Could you check a few things on this model? Use its own coordinates, in mm. A direction names the side the tool comes from. Give positions to 0.01 mm unless a question says otherwise; leave off trailing zeros. Loops run counter-clockwise (first coordinate to the right, second up) from the corner with the lowest first, then second, coordinate; pieces in that order, holes last. Notation, with made-up numbers: (7, 9.5) - (29, 9.5) arc R10 ccw to (29, 16.5) - close; hole circle Ø5 at (63, 2.5). An arc over 180 degrees is marked (long way). Write each question's results on one line, items separated by ' | '. Start each with the question number.
1) If I drill on probe 1 along Y at (x, z) = (0, -2.25); probe 2 along Y at (x, z) = (4.5, -1.75); probe 3 along Y at (x, z) = (0, -15.25), over which ranges is the centre line in solid material (lowest first)? Write a range as [from, to].
2) I'm going to push flat-ended pins straight in: pin 1 (3.5 mm diameter, centred on x = -1, z = -13.5, fed in from -Y); pin 2 (4 mm diameter, centred on y = 5.5, z = -5.5, fed in from -X); pin 3 (1.5 mm diameter, centred on y = 4, z = -3, fed in from +X); pin 4 (9 mm diameter, centred on x = -2.5, y = 1, fed in from -Z). Where does each tip first touch, or does it pass through?
3) I want a section at A-A, the plane z = -6. Write out the boundary of the cut face in (x, y), and give its area (3 significant figures).
4) On a 3-axis mill with a long thin cutter (end or side, diameter ignored), from which of +Z, -Z, +X, -X, +Y, -Y can I reach the whole of each face in a straight line? I mean faces 4 (the face through (5.04, 5.08, -15)), 5 (the face through (0, 2, -6.5)), 6 (the face through (4, -6, 1)). Say none if no direction works.
5) If we mould it in two halves opening along X, with no side actions, what happens to faces 1 (the face through (-0.1, 1.56, -3.03)), 2 (the face through (7.327, -4.309, -13.521)), 3 (the face through (0, -8.5, -14))? For each: +X half, -X half, draft (parallel to the pull), parting line (faces both ways), or undercut.
6) I want a section at B-B, the plane z = -12.75. Write out the boundary of the cut face in (x, y), and give its area (3 significant figures).
from build123d import *

# Parameters (mm, degrees)
SKETCH1_R          = 9
EXTRUDE1_DEPTH     = 2
SKETCH4_R          = 7
EXTRUDE2_DEPTH     = 16
SKETCH2_R          = 5.5
CUT_EXTRUDE1_DEPTH = 10
SKETCH3_R          = 8.25
SKETCH3_R_2        = 7
CUT_EXTRUDE2_DEPTH = 1
SKETCH5_R          = 5
EXTRUDE3_DEPTH     = 8.5
SKETCH6_R          = 0.45
CUT_EXTRUDE3_DEPTH = 7
CHAMFER2_SIZE      = 0.15
CHAMFER1_SIZE      = 0.2
SKETCH7_R          = 5.5
CUT_EXTRUDE4_DEPTH = 1
CHAMFER3_SIZE      = 0.5
EXTRUDE4_DEPTH     = 3


with BuildPart() as part:
    # Sketch1 → Extrude1 (new body)
    with BuildSketch(Plane.XY):
        Circle(SKETCH1_R)
    extrude(amount=EXTRUDE1_DEPTH)

    # Sketch4 → Extrude2 (add)
    with BuildSketch(Plane(origin=(0, 0, 0), x_dir=(-1, 0, 0), z_dir=(0, 0, -1))):
        Circle(SKETCH4_R)
    extrude(amount=EXTRUDE2_DEPTH)

    # Sketch2 → Cut-Extrude1 (cut)
    with BuildSketch(Plane.XY.offset(2)):
        Circle(SKETCH2_R)
    extrude(amount=-CUT_EXTRUDE1_DEPTH, mode=Mode.SUBTRACT)

    # Sketch3 → Cut-Extrude2 (cut)
    with BuildSketch(Plane(origin=(0, 0, 0), x_dir=(-1, 0, 0), z_dir=(0, 0, -1))):
        Circle(SKETCH3_R)
        Circle(SKETCH3_R_2, mode=Mode.SUBTRACT)
    extrude(amount=-CUT_EXTRUDE2_DEPTH, mode=Mode.SUBTRACT)

    # Sketch5 → Extrude3 (add)
    with BuildSketch(Plane.XY.offset(-8)):
        Circle(SKETCH5_R)
    extrude(amount=EXTRUDE3_DEPTH)

    # Sketch6 → Cut-Extrude3 (cut)
    with BuildSketch(Plane.XY.offset(0.5)):
        with Locations((0, 2)):
            Circle(SKETCH6_R)
        with Locations((0, -2)):
            Circle(SKETCH6_R)
        with Locations((2, 0)):
            Circle(SKETCH6_R)
        with Locations((-2, 0)):
            Circle(SKETCH6_R)
    extrude(amount=-CUT_EXTRUDE3_DEPTH, mode=Mode.SUBTRACT)

    # Chamfer2
    chamfer2_edges = [part.edges().sort_by_distance(p)[0] for p in [
        (-5, 0, 0.5),
        (-0.45, 2, 0.5),
        (-0.45, -2, 0.5),
        (1.55, 0, 0.5),
        (-2.45, 0, 0.5),
    ]]
    chamfer(chamfer2_edges, length=CHAMFER2_SIZE)

    # Chamfer1
    chamfer1_edges = [part.edges().sort_by_distance(p)[0] for p in [
        (-5.5, 0, 2),
        (-9, 0, 2),
    ]]
    chamfer(chamfer1_edges, length=CHAMFER1_SIZE)

    # Sketch7 → Cut-Extrude4 (cut)
    with BuildSketch(Plane(origin=(0, 0, -16), x_dir=(-1, 0, 0), z_dir=(0, 0, -1))):
        Circle(SKETCH7_R)
    extrude(amount=-CUT_EXTRUDE4_DEPTH, mode=Mode.SUBTRACT)

    # Chamfer3
    chamfer3_edges = [part.edges().sort_by_distance(p)[0] for p in [
        (7, 0, -16),
    ]]
    chamfer(chamfer3_edges, length=CHAMFER3_SIZE)

    # Sketch8 → Extrude4 (add)
    with BuildSketch(Plane(origin=(0, 0, -15), x_dir=(-1, 0, 0), z_dir=(0, 0, -1))):
        Polygon((-4.907477288, 8.5), (4.907477288, 8.5), (9.814954576, 0), (4.907477288, -8.5), (-4.907477288, -8.5), (-9.814954576, 0), align=None)
    extrude(amount=-EXTRUDE4_DEPTH)


solid = part.part
Answers:
1) probe 1: y = [-7, -5.5], [-5, -2.45], [-1.55, 1.55], [2.45, 5], [5.5, 7] | probe 2: y = [-5.36, -3.16], [-2.18, 2.18], [3.16, 5.36] | probe 3: y = [-7, -5.5], [5.5, 7]
2) pin 1: stops at y = -8.5 | pin 2: stops at x = -6.06 | pin 3: stops at x = 6.2 | pin 4: stops at z = -16
3) outline: circle Ø14 at (0, 0); circle Ø10 at (0, 0); hole circle Ø11 at (0, 0); hole circle Ø0.9 at (-2, 0); hole circle Ø0.9 at (0, -2); hole circle Ø0.9 at (0, 2); hole circle Ø0.9 at (2, 0) | area: 135 mm2
4) face 4: -Z | face 5: +Z | face 6: none
5) face 1: undercut | face 2: +X half | face 3: draft
6) outline: (-9.81, 0) - (-4.91, -8.5) - (4.91, -8.5) - (9.81, 0) - (4.91, 8.5) - (-4.91, 8.5) - close | area: 250 mm2
